Design review of the part built by this model. Coordinates are the model's own, in mm. Face numbers are marked on the shaded views. Give positions to 0.01 mm unless a question says otherwise; leave off trailing zeros. Order: outer loops, then holes, each group sorted by start corner. A loop starts at its lowest first (then second) coordinate and runs counter-clockwise, first axis right, second up. Notation, with made-up numbers: M -37.75,-25 L 0.25,-25 A11 ccw 0.25,-5 Z; hole C -15.5,-35.5 d6. An arc over 180 degrees is marked long. Answer as a JSON object with one key per item and string values.
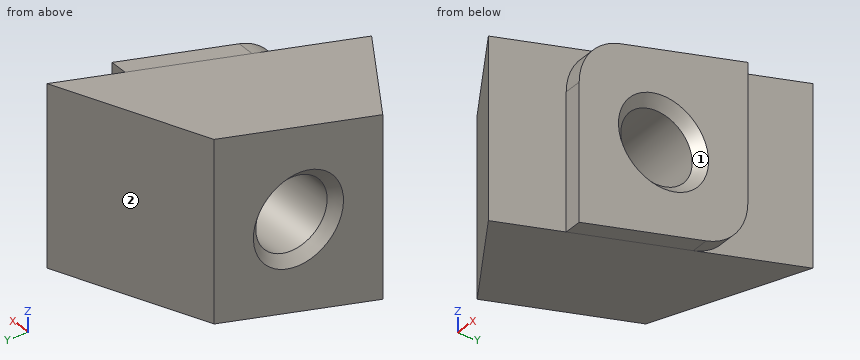
from build123d import *

# Parameters (mm, degrees)
EXTRUDE1_DEPTH        = 0.8
EXTRUDE2_DEPTH        = 5.5
DRAFT1_ANGLE          = -33.206570315
DRAFT2_ANGLE          = -33.206570315
M4_TAPPED_HOLE1_D     = 3.3
M4_TAPPED_HOLE1_DEPTH = 6.3
CHAMFER1_SIZE         = 0.433


with BuildPart() as part:
    # Sketch1 → Extrude1 (new body)
    with BuildSketch(Plane(origin=(0, 0, 0), x_dir=(0, 0, -1), z_dir=(1, 0, 0))):
        with BuildLine():
            Line((1.101052702, 3.9), (-5.186106572, 3.9))
            Line((-5.186106572, 3.9), (-3.612459851, -1.972929517))
            ThreePointArc((-3.612459851, -1.972929517), (-2.683832418, -3.362718685), (-1.101052702, -3.9))
            Line((-1.101052702, -3.9), (5.186106572, -3.9))
            Line((5.186106572, -3.9), (3.612459851, 1.972929517))
            ThreePointArc((3.612459851, 1.972929517), (2.683832418, 3.362718685), (1.101052702, 3.9))
        make_face()
    extrude(amount=-EXTRUDE1_DEPTH)

    # Sketch2 → Extrude2 (add)
    with BuildSketch(Plane.ZY.offset(0.8)):
        with BuildLine():
            Line((2.131485778, -7.5), (-6.150723665, -7.5))
            add(Edge.make_bspline(
                [(-2.131485778, 7.5), (-3.471231741, 2.5), (-4.810977703, -2.5), (-6.150723665, -7.5)],
                knots=[0, 0, 0, 0, 1, 1, 1, 1], degree=3))
            Line((-2.131485778, 7.5), (6.150723665, 7.5))
            add(Edge.make_bspline(
                [(2.131485778, -7.5), (3.471231741, -2.5), (4.810977703, 2.5), (6.150723665, 7.5)],
                knots=[0, 0, 0, 0, 1, 1, 1, 1], degree=3))
        make_face()
    extrude(amount=EXTRUDE2_DEPTH)

    # Draft1
    draft1_faces = [part.faces().sort_by_distance(p)[0] for p in [
        (-3.55, 7.5, 2.009618943),
    ]]
    draft(draft1_faces, Plane(origin=(-0.8, 0, 4.141104722), x_dir=(0, 0, 1), z_dir=(1, 0, 0)), DRAFT1_ANGLE)

    # Draft2
    draft2_faces = [part.faces().sort_by_distance(p)[0] for p in [
        (-3.55, -7.5, -2.009618943),
    ]]
    draft(draft2_faces, Plane(origin=(-0.8, 0, 4.141104722), x_dir=(0, 0, 1), z_dir=(1, 0, 0)), DRAFT2_ANGLE)

    # M4 Tapped Hole1
    with Locations(Plane.ZY.offset(6.3)):
        with Locations((0, 0)):
            Hole(M4_TAPPED_HOLE1_D / 2, depth=M4_TAPPED_HOLE1_DEPTH)

    # Chamfer1
    chamfer1_edges = [part.edges().sort_by_distance(p)[0] for p in [
        (-6.3, 0, 1.65),
        (0, 0, 1.65),
    ]]
    chamfer(chamfer1_edges, length=CHAMFER1_SIZE)


solid = part.part
(1) We need section B-B (x = -0.25). Write out the cut boundary in (y, z).
Checked values:
{"outline": "M -3.9,-5.19 L 1.97,-3.61 A2.6 ccw 3.9,-1.1 L 3.9,5.19 L -1.97,3.61 A2.6 ccw -3.9,1.1 Z; hole C 0,0 d3.67"}
(2) We need section A-A (z = 0). Write out the cut boundary in (x, y), plus the area to 3 significant figures.
Checked values:
{"outline": "M -6.3,-3.9 L -0.8,-7.5 L -0.8,-3.9 L 0,-3.9 L 0,-2.08 L -0.43,-1.65 L -5.87,-1.65 L -6.3,-2.08 Z; M -6.3,2.08 L -5.87,1.65 L -0.43,1.65 L 0,2.08 L 0,3.9 L -0.8,3.9 L -0.8,7.5 L -6.3,3.9 Z", "area": "47.8 mm^2"}
(3) Draft analysis for pull direction Z (two halves, no side actions). For the marked faces 1 and 2, state which applies: +Z half, -Z half, draft (parallel to the pull), parting line (faces both ways), or undercut.
Checked values:
{"face 1": "undercut", "face 2": "draft"}
(4) Insertion check: pin 1 (0.6 mm diameter, centred on x = 0, z = -2.5, fed in from -Y); pin 2 (4 mm diameter, centred on y = 0, z = 0, fed in from -X); pin 3 (1 mm diameter, centred on x = -4.5, z = -4, fed in from -Y). Each pin has a flat end and moves straight along its axis. Give the tip position at first contact, or say it passes through.
Checked values:
{"pin 1": "stops at y = -3.9", "pin 2": "stops at x = -6.22", "pin 3": "stops at y = -5.41"}
(5) To check wall thickness, follow L1, parallel to Y at x = -2, z = 0; L2, parallel to Y at x = -5.75, z = 0.5; L3, parallel to X at y = 6, z = 4.5. State the ranges of each line that lie inside material, in increasing order. Write a range as from..to.
Checked values:
{"L1": "y = -6.71..-1.65, 1.65..6.71", "L2": "y = -4.26..-1.57, 1.57..4.26", "L3": "x = -3.09..-0.8"}
